Could you check a few things on this model? Use its own coordinates, in mm. Give positions to 0.01 mm unless a question says otherwise; leave off trailing zeros. Loops run counter-clockwise (first coordinate to the right, second up) from the corner with the lowest first, then second, coordinate; pieces in that order, holes last. Notation, with made-up numbers: M 76,22 L 117,22 A19 ccw 117,50 Z; hole C 7,58 d7. An arc over 180 degrees is marked long. Answer in a Markdown table with one row per item. Add a question column.
1. I'm going to push flat-ended pins straight in: pin 1 Ø8 at (x, z) = (96.5, -17.5) entering from +Y; pin 2 Ø6 at (x, z) = (67.5, -12) entering from -Y; pin 3 Ø4 at (y, z) = (-41, -63.5) entering from -X. Where does each tip first touch, or does it pass through?
2. If we section it at C-C on y = -71.5: List the corners of the cut face in (x, z) for me, then the cut area to 3 significant figures.
3. If we section it at B-B on x = 106: List the corners of the cut face in (y, z) for me, then the cut area to 3 significant figures.
4. I need wall thicknesses on line 1 along Y through (x, z) = (91, -42); line 2 along X through (y, z) = (-45.5, -67); line 3 along X through (y, z) = (-3.5, -4.5). Which ranges of each line are inside material? Lowest first, please. Write a range as from..to.
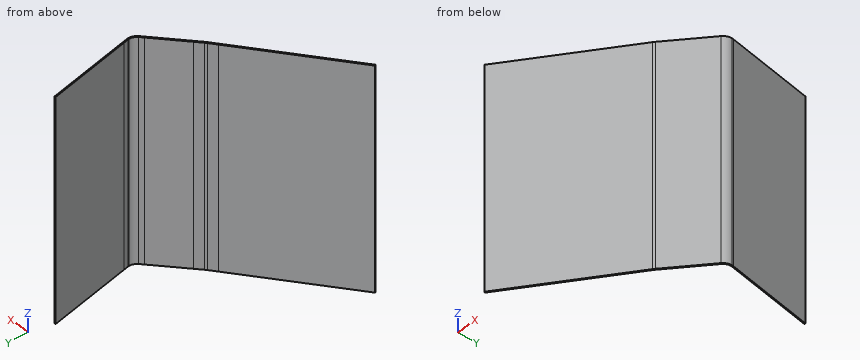
Autodesk Inventor part; units mm, degrees
ref_plane "YZ Plane" through (0, 0, 0) normal (1, 0, 0) x (0, 1, 0)
ref_plane "XZ Plane" through (0, 0, 0) normal (0, 1, 0) x (-1, 0, 0)
ref_plane "XY Plane" through (0, 0, 0) normal (0, 0, 1) x (1, 0, 0)
sketch "スケッチ1" plane through (0, 0, 0) normal (0, 0, 1) x (1, 0, 0)
  line L0 (109.2087, 3) -> (109.2087, 0)
  line L1 (109.2087, -3) -> (109.2087, 0)
  circle A0 centre (111.885, -36) radius 4
  circle A1 centre (47.8869, -85.25) radius 4
  line L2 (109.2087, 3) -> (115.8267, -35.3193)
  line L3 (116.3194, -35.2342) -> (108.7087, 8.833)
  line L4 (108.7087, 8.833) -> (108.7087, 0)
  circle A2 centre (111.885, -36) radius 4.5
  line L5 (109.2087, 3) -> (109.7014, 3.0851)
  circle A3 centre (88.5017, -43.0436) radius 13.85
  line L6 (96.7244, -54.1885) -> (50.2617, -88.4688)
  line L7 (114.4855, -39.0393) -> (97.5058, -53.5673)
  line L8 (114.8106, -39.4192) -> (97.8309, -53.9472)
  circle A4 centre (88.5017, -43.0436) radius 14.35
  line L9 (97.0213, -54.5908) -> (50.5586, -88.8711)
  line L10 (50.5586, -88.8711) -> (50.2617, -88.4688)
  point P0 (0, 0)
  dimension "d0" = 0.5
  dimension "d1" = 0.5
  dimension "d2" = 0.5
  dimension "d3" = 0.5
  dimension "d4" = 0.5
extrude "押し出し1" add sketch "スケッチ1" against normal blind 98.8 contours A0 L2 A2 L7 | L2 L5 L3 A2 | A2 L8 A4 L7 | A4 L6 A3 L7 | L9 L10 L6 A4 picked at (113.6675, -39.86) picked at (95.0962, -55.5046)
properties part number "機体ケツ防護カバーver2" material "ポリカーボネート、クリア"
Results:
| question | item | result |
|---|---|---|
| 1 | pin 1 | y = -51.01 |
| 1 | pin 2 | y = -78.59 |
| 1 | pin 3 | x = 109.86 |
| 2 | outline | M 73.26,-98.8 L 74.1,-98.8 L 74.1,0 L 73.26,0 Z |
| 2 | area | 83.2 mm2 |
| 3 | outline | M -46.96,-98.8 L -46.3,-98.8 L -46.3,0 L -46.96,0 Z |
| 3 | area | 65.0 mm2 |
| 4 | line 1 | -59.03..-58.41 |
| 4 | line 2 | 106.93..107.7 |
| 4 | line 3 | 110.33..110.84 |
